```python
from build123d import *

# Parameters (mm, degrees)
BOSS_EXTRUDE1_DEPTH = 13.2334
BOSS_EXTRUDE2_DEPTH = 14.605
CUT_EXTRUDE1_DEPTH  = 14.36116


with BuildPart() as part:
    # Sketch1 → Boss-Extrude1 (new body)
    with BuildSketch(Plane.XY):
        Polygon((-1.142068777, 0), (1.142068777, 0), (1.397, 14.605), (-1.397, 14.605), align=None)
    extrude(amount=BOSS_EXTRUDE1_DEPTH)

    # Sketch2 → Boss-Extrude2 (add)
    with BuildSketch(Plane.XZ):
        Polygon((-0.8001, 13.2334), (0.8001, 13.2334), (0.23114, 13.79728), (-0.23368, 13.79728), align=None)
    boss_extrude2 = extrude(amount=-BOSS_EXTRUDE2_DEPTH)

    # Mirror1: Boss-Extrude2 across plane
    add(boss_extrude2.mirror(Plane.XY.offset(6.6167)))

    # Sketch3 → Cut-Extrude1 (cut)
    with BuildSketch(Plane.XY.offset(13.79728)):
        Polygon((-1.243534982, 5.812994982), (-0.23368, 4.8006), (-0.23368, 4.3434), (-1.200976725, 3.374834107), align=None)
        Polygon((1.243534982, 5.812994982), (0.23114, 4.8006), (0.23114, 4.3434), (1.200976725, 3.374834107), align=None)
    extrude(amount=-CUT_EXTRUDE1_DEPTH, mode=Mode.SUBTRACT)


solid = part.part
```
Check sheet for the modelled part. Datum: model origin and axes. Units: mm. A direction names the side the tool comes from. Round coordinates to 2 decimals unless told otherwise and drop trailing zeros. Order: outer loops, then holes, each group sorted by start corner. A loop starts at its lowest first (then second) coordinate and runs counter-clockwise, first axis right, second up. Notation, with made-up numbers: (18, 12.5) -> (46, 12.5) arc R25 ccw to (46, 35.5) -> close; hole circle Ø1 at (-17, 49.25). An arc over 180 degrees is marked (long way). One line per item, written item: value. Start each with the question number.
Q1. Set-up check for faces 4 (the face through (-0.711, 3.866, 6.717)), 5 (the face through (0.709, 3.866, 6.717)): record each of +Z, -Z, +X, -X, +Y, -Y from which the full face is reachable in a straight line by a thin tool's end or side.
Q2. Gauge pin test, flat ends, axial feed: pin 1 Ø1.5 at (y, z) = (8, 11.5) entering from -X; pin 2 Ø4 at (y, z) = (11, 8) entering from -X; pin 3 Ø1.5 at (y, z) = (1.5, 5) entering from -X. Record the tip position at first contact, or that the pin passes through.
Q3. Mould release check, pull along Y, two halves, no side actions. Record for faces 1 (the face through (-0.746, 5.314, 6.717)), 2 (the face through (0, 14.605, 7)), 3 (the face through (0, 0, 7)): pulls with the +Y half, pulls with the -Y half, needs draft (parallel to the pull), parting line crosses it, or undercut.
Q4. Thickness scan on line 1 (Y direction, x = -0.8, z = 12) (3 decimals); line 2 (Z direction, x = 0.85, y = 2.5); line 3 (Y direction, x = -0.45, z = 11.5) (3 decimals). Record the ranges inside material, lowest first.
Q5. Cross-section at C-C (y = 7.75). Record the boundary of the cut face in (x, z).
Q6. Cross-section at A-A (x = 0.6). Record the boundary of the cut face in (y, z) (3 decimals).
Q7. Cross-section at B-B (z = 4). Record the boundary of the cut face in (x, y) (3 decimals), and give its area (3 significant figures).
Completed:
1. face 4: +Z, -Z, -X
1. face 5: +Z, -Z, +X
2. pin 1: stops at x = -1.29
2. pin 2: stops at x = -1.37
2. pin 3: stops at x = -1.18
3. face 1: undercut
3. face 2: pulls with the +Y half
3. face 3: pulls with the -Y half
4. line 1: y = 0 to 3.776, 5.368 to 14.605
4. line 2: z = 0 to 13.23
4. line 3: y = 0 to 4.127, 5.017 to 14.605
5. outline: (-1.28, 0) -> (-0.8, 0) -> (-0.23, -0.56) -> (0.23, -0.56) -> (0.8, 0) -> (1.28, 0) -> (1.28, 13.23) -> (0.8, 13.23) -> (0.23, 13.8) -> (-0.23, 13.8) -> (-0.8, 13.23) -> (-1.28, 13.23) -> close
6. outline: (0, -0.198) -> (3.975, -0.198) -> (3.975, 13.432) -> (0, 13.432) -> close; (5.169, -0.198) -> (14.605, -0.198) -> (14.605, 13.432) -> (5.169, 13.432) -> close
7. outline: (-1.397, 14.605) -> (-1.244, 5.813) -> (-0.234, 4.801) -> (-0.234, 4.343) -> (-1.201, 3.375) -> (-1.142, 0) -> (1.142, 0) -> (1.201, 3.375) -> (0.231, 4.343) -> (0.231, 4.801) -> (1.244, 5.813) -> (1.397, 14.605) -> close
7. area: 34.2 mm²
